Input: part model. Units: mm. Frame: model coordinates. A direction names the side the tool comes from. Coordinates: 2 decimals unless noted, no trailing zeros. Write each loop counter-clockwise with the first axis right and the second up, starting at its lowest first coordinate (ties: lowest second). Pieces come first, ordered by that corner, then holes.
1) Section query A-A (x = 0). Output: boundary loops of the cut face in (y, z).
2) Line query: L1, parallel to X at y = -0.25, z = 37.5; L2, parallel to X at y = 2, z = 5.5; L3, parallel to Y at x = 0, z = 35. Output: solid intervals per line, ascending.
3) Set-up query: faces 5 (the cylindrical face through (-0.867, -3.905, 31.154)), 6 (the cylindrical face through (8.43, -0.02, 4.96)), 7 (the cylindrical face through (-10.3, 2, 2.4)), 8 (the flat face through (0, 2.5, 1)). Return all of +Z, -Z, +X, -X, +Y, -Y with unobstructed straight access to the full face (end or side cutting, diameter ignored); none if empty.
4) Section query B-B (z = 10.5). Output: boundary loops of the cut face in (x, y), then the cut area to 3 significant figures.
5) Pin query (flat end, axial travel): pin 1 Ø4 at (x, z) = (3, 17) entering from +Y; pin 2 Ø1.5 at (x, z) = (-4.5, 5) entering from -Y; pin 3 Ø1.8 at (x, y) = (1, 3.5) entering from -Z; pin 4 Ø8 at (x, z) = (-2.5, 11.5) entering from -Y. Return the tip coordinate at first contact, or that it passes through.
6) Section query D-D (z = 4). Output: boundary loops of the cut face in (x, y).
7) Draft query along Z for faces 1 (the flat face through (0, 0, 7)), 2 (the flat face through (9, 0, 20)), 3 (the flat face through (0, -4, 18)), 4 (the flat face through (-12.5, 0, 10)). Return one class per face: pulls with the +Z half, pulls with the -Z half, needs draft (parallel to the pull), parting line crosses it, or undercut.
8) Section query C-C (y = 0). Output: boundary loops of the cut face in (x, z).
from build123d import *

# Parameters (mm, degrees)
SKETCH006_W     = 25
SKETCH006_H     = 5
PAD_DEPTH       = 20
SKETCH_R        = 6
PAD001_DEPTH    = 24
SKETCH001_R     = 4
POCKET001_DEPTH = 22
POCKET002_DEPTH = 5
POCKET003_DEPTH = 1


with BuildPart() as part:
    # Sketch006 → Pad (new body)
    with BuildSketch(Plane.XY):
        Rectangle(SKETCH006_W, SKETCH006_H)
    extrude(amount=PAD_DEPTH)

    # Sketch (on Face6 of Pad) → Pad001 (join)
    with BuildSketch(Plane.XY.offset(18)):
        Circle(SKETCH_R)
    extrude(amount=PAD001_DEPTH)

    # Sketch001 (on Face11 of Pad001) → Pocket001 (cut)
    with BuildSketch(Plane.XY.offset(42)):
        Circle(SKETCH001_R)
    extrude(amount=-POCKET001_DEPTH, mode=Mode.SUBTRACT)

    # Sketch009 (on Face9 of Pocket001) → Pocket002 (cut)
    with BuildSketch(Plane.XZ.offset(2.5)):
        with BuildLine():
            ThreePointArc((-6.430284, 7), (-8.430284, 5), (-6.430284, 3))
            Line((-6.430284, 3), (6.430284, 3))
            ThreePointArc((6.430284, 3), (8.430284, 5), (6.430284, 7))
            Line((-6.430284, 7), (6.430284, 7))
        make_face()
    extrude(amount=-POCKET002_DEPTH, mode=Mode.SUBTRACT)

    # Sketch010 (on Face13 of Pocket002) → Pocket003 (cut)
    with BuildSketch(Plane.XZ.offset(2.5)):
        with BuildLine():
            Line((-7.41661, 17.549025), (7.41661, 17.549025))
            ThreePointArc((11.41661, 13.549025), (10.245037, 16.377452), (7.41661, 17.549025))
            Line((11.41661, 13.549025), (11.41661, 5.173753))
            ThreePointArc((7.41661, 1.173753), (10.245037, 2.345326), (11.41661, 5.173753))
            Line((7.41661, 1.173753), (-7.41661, 1.173753))
            ThreePointArc((-11.41661, 5.173753), (-10.245037, 2.345326), (-7.41661, 1.173753))
            Line((-11.41661, 5.173753), (-11.41661, 13.549025))
            ThreePointArc((-7.41661, 17.549025), (-10.245037, 16.377452), (-11.41661, 13.549025))
        make_face()
    pocket003 = extrude(amount=-POCKET003_DEPTH, mode=Mode.SUBTRACT)

    # Mirrored: Pocket003 across XZ
    add(pocket003.mirror(Plane.XZ), mode=Mode.SUBTRACT)


solid = part.part
Answer:
1. outline: (-6, 18) - (-2.5, 18) - (-2.5, 17.55) - (-1.5, 17.55) - (-1.5, 7) - (1.5, 7) - (1.5, 17.55) - (2.5, 17.55) - (2.5, 18) - (6, 18) - (6, 42) - (4, 42) - (4, 20) - (-4, 20) - (-4, 42) - (-6, 42) - close; (-2.5, 0) - (2.5, 0) - (2.5, 1.17) - (1.5, 1.17) - (1.5, 3) - (-1.5, 3) - (-1.5, 1.17) - (-2.5, 1.17) - close
2. L1: x = -5.99 to -3.99, 3.99 to 5.99
2. L2: x = -12.5 to -11.42, 11.42 to 12.5
2. L3: y = -6 to -4, 4 to 6
3. face 5: +Z
3. face 6: +Y, -Y
3. face 7: +Y
3. face 8: -Z, +Y
4. outline: (-12.5, -2.5) - (-11.42, -2.5) - (-11.42, -1.5) - (11.42, -1.5) - (11.42, -2.5) - (12.5, -2.5) - (12.5, 2.5) - (11.42, 2.5) - (11.42, 1.5) - (-11.42, 1.5) - (-11.42, 2.5) - (-12.5, 2.5) - close
4. area: 79.3 mm2
5. pin 1: stops at y = 5.86
5. pin 2: passes through
5. pin 3: stops at z = 18
5. pin 4: stops at y = -1.5
6. outline: (-12.5, -2.5) - (-11.24, -2.5) - (-11.24, -1.5) - (-8.16, -1.5) - (-8.16, 1.5) - (-11.24, 1.5) - (-11.24, 2.5) - (-12.5, 2.5) - close; (8.16, -1.5) - (11.24, -1.5) - (11.24, -2.5) - (12.5, -2.5) - (12.5, 2.5) - (11.24, 2.5) - (11.24, 1.5) - (8.16, 1.5) - close
7. face 1: undercut
7. face 2: pulls with the +Z half
7. face 3: pulls with the -Z half
7. face 4: needs draft
8. outline: (-12.5, 0) - (12.5, 0) - (12.5, 20) - (6, 20) - (6, 42) - (4, 42) - (4, 20) - (-4, 20) - (-4, 42) - (-6, 42) - (-6, 20) - (-12.5, 20) - close; hole (-6.43, 3) - (6.43, 3) arc R2 ccw to (6.43, 7) - (-6.43, 7) arc R2 ccw to start
